```python
from build123d import *

# Parameters (mm, degrees)
SKETCH1_W           = 19
SKETCH1_H           = 62
BOSS_EXTRUDE1_DEPTH = 5


with BuildPart() as part:
    # Sketch1 → Boss-Extrude1 (new body)
    with BuildSketch(Plane(origin=(0, 0, 0), x_dir=(1, 0, 0), z_dir=(0, 1, 0))):
        Polygon((-1.543955144, 19.039548023), (-1.543955144, -0.960451977), (5.956044856, -0.960451977), (5.956044856, -5.960451977), (10.956044856, -5.960451977), (10.956044856, -0.960451977), (13.956044856, -0.960451977), (13.956044856, 2.039548023), (12.456044856, 2.039548023), (12.456044856, 4.539548023), (13.956044856, 4.539548023), (13.956044856, 9.039548023), (17.956044856, 9.039548023), (17.956044856, 4.539548023), (19.456044856, 4.539548023), (19.456044856, 2.039548023), (17.956044856, 2.039548023), (17.956044856, -0.960451977), (20.956044856, -0.960451977), (20.956044856, -5.960451977), (25.956044856, -5.960451977), (25.956044856, -0.960451977), (33.456044856, -0.960451977), (33.456044856, 19.039548023), (33.456044856, 81.039548023), (33.456044856, 101.039548023), (25.956044856, 101.039548023), (25.956044856, 106.039548023), (20.956044856, 106.039548023), (20.956044856, 101.039548023), (17.956044856, 101.039548023), (17.956044856, 98.039548023), (19.456044856, 98.039548023), (19.456044856, 95.539548023), (17.956044856, 95.539548023), (17.956044856, 91.039548023), (13.956044856, 91.039548023), (13.956044856, 95.539548023), (12.456044856, 95.539548023), (12.456044856, 98.039548023), (13.956044856, 98.039548023), (13.956044856, 101.039548023), (10.956044856, 101.039548023), (10.956044856, 106.039548023), (5.956044856, 106.039548023), (5.956044856, 101.039548023), (-1.543955144, 101.039548023), (-1.543955144, 81.039548023), align=None)
        with Locations((15.956044856, 50.039548023)):
            Rectangle(SKETCH1_W, SKETCH1_H, mode=Mode.SUBTRACT)
    extrude(amount=BOSS_EXTRUDE1_DEPTH)


solid = part.part
```
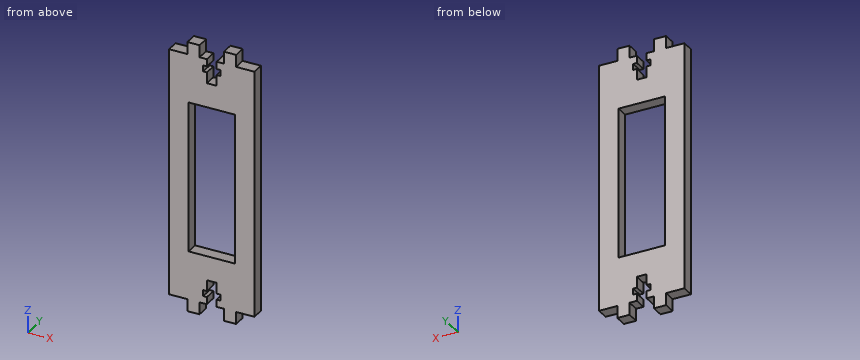
The listing builds one solid part. Answer for the finished solid, in the listing's coordinates (mm). Give positions to 0.01 mm unless a question says otherwise; leave off trailing zeros. Loops run counter-clockwise (first coordinate to the right, second up) from the corner with the lowest first, then second, coordinate; pieces in that order, holes last. Notation, with made-up numbers: (-33.5, 66) - (-17.5, 66) arc R10 cw to (-17.5, 70) - close; hole circle Ø4 at (33, 13). An arc over 180 degrees is marked (long way). Return JSON: item names as keys, results as strings. Group by question number.
1. Given pin 1 Ø1.5 at (x, y) = (28, 1.5) entering from +Z; pin 2 Ø1.6 at (x, y) = (19, 3.5) entering from -Z; pin 3 Ø2 at (x, y) = (15.5, 2.5) entering from -Z, each flat-ended and moving along its own axis, determine where each tip first touches the part or whether it passes through.
2. Straight lines are drawn through the part: line 1 (X direction, y = 1.55, z = -19.5); line 2 (Z direction, x = 11, y = 0.9); line 3 (Z direction, x = 16, y = 4.25). For each, find the intervals that lie inside material, in ascending order. Write a range as [from, to].
3. Find section C-C (x = 27). Write down the section's boundary in (y, z), then the cut area to 3 significant figures.
4. Find section B-B (x = 16). Write down the section's boundary in (y, z), then the cut area to 4 significant figures.
5. Find section A-A (z = -6.5). Write down the section's boundary in (x, y).
Verdict:
{
 "1": {"pin 1": "stops at z = 0.96", "pin 2": "stops at z = -101.04", "pin 3": "stops at z = -91.04"},
 "2": {"line 1": "x = [-1.54, 6.46], [25.46, 33.46]", "line 2": "z = [-101.04, -81.04], [-19.04, 0.96]", "line 3": "z = [-91.04, -81.04], [-19.04, -9.04]"},
 "3": {"outline": "(0, -101.04) - (5, -101.04) - (5, 0.96) - (0, 0.96) - close", "area": "510 mm^2"},
 "4": {"outline": "(0, -91.04) - (5, -91.04) - (5, -81.04) - (0, -81.04) - close; (0, -19.04) - (5, -19.04) - (5, -9.04) - (0, -9.04) - close", "area": "100.0 mm^2"},
 "5": {"outline": "(-1.54, 0) - (13.96, 0) - (13.96, 5) - (-1.54, 5) - close; (17.96, 0) - (33.46, 0) - (33.46, 5) - (17.96, 5) - close"}
}
